Input: dimensioned drawing with shaded views. Units: mm. Origin: part minimum x, y, z. Give positions to 0.01 mm unless a question says otherwise; leave off trailing zeros. Write each loop counter-clockwise with the first axis right and the second up, starting at its lowest first coordinate (ties: lowest second). Pieces come first, ordered by that corner, then holes.
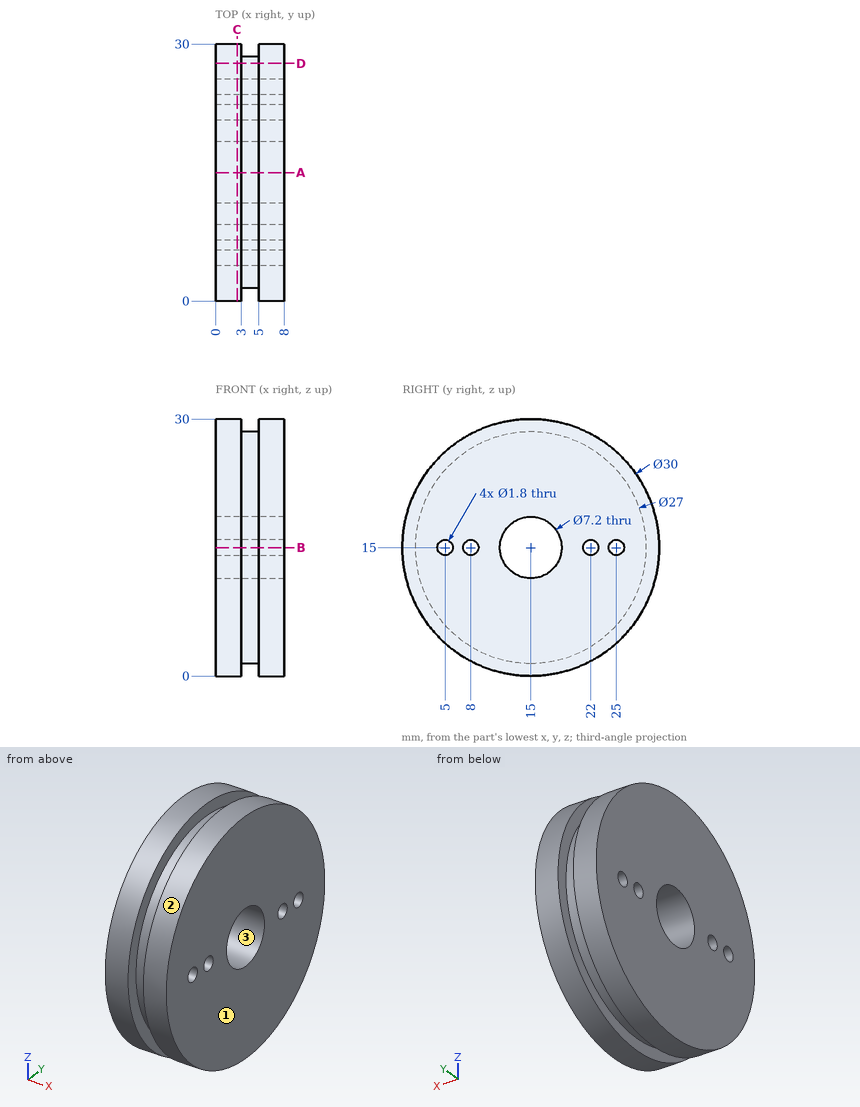
Item 1: Section A-A, the plane y = 15. Return the cut outline in (x, z), plus the area to 3 significant figures.
Found:
outline: (0, 0) - (3, 0) - (3, 1.5) - (5, 1.5) - (5, 0) - (8, 0) - (8, 11.4) - (0, 11.4) - close; (0, 18.6) - (8, 18.6) - (8, 30) - (5, 30) - (5, 28.5) - (3, 28.5) - (3, 30) - (0, 30) - close
area: 176 mm2
Item 2: Pull-direction query (Z, two-part tool) for the marked faces 1, 2 and 3; classes: +Z half, -Z half, draft (parallel to the pull), parting line (faces both ways), or undercut.
Found:
face 1: draft
face 2: parting line
face 3: undercut
Item 3: Section C-C, the plane x = 2.5. Return the cut outline in (y, z), plus the area to 3 significant figures.
Found:
outline: circle Ø30 at (15, 15); hole circle Ø1.8 at (5, 15); hole circle Ø1.8 at (8, 15); hole circle Ø7.2 at (15, 15); hole circle Ø1.8 at (22, 15); hole circle Ø1.8 at (25, 15)
area: 656 mm2
Item 4: Section D-D, the plane y = 27.75. Return the cut outline in (x, z), plus the area to 3 significant figures.
Found:
outline: (0, 7.1) - (3, 7.1) - (3, 10.56) - (5, 10.56) - (5, 7.1) - (8, 7.1) - (8, 22.9) - (5, 22.9) - (5, 19.44) - (3, 19.44) - (3, 22.9) - (0, 22.9) - close
area: 113 mm2
Item 5: Line query: L1, parallel to Y at x = 6, z = 15; L2, parallel to Y at x = 4.25, z = 15; L3, parallel to Z at x = 7, y = 15. Output: solid intervals per line, ascending.
Found:
L1: y = 0 to 4.1, 5.9 to 7.1, 8.9 to 11.4, 18.6 to 21.1, 22.9 to 24.1, 25.9 to 30
L2: y = 1.5 to 4.1, 5.9 to 7.1, 8.9 to 11.4, 18.6 to 21.1, 22.9 to 24.1, 25.9 to 28.5
L3: z = 0 to 11.4, 18.6 to 30
Item 6: Pin query (flat end, axial travel): pin 1 Ø1.4 at (y, z) = (25, 15) entering from +X; pin 2 Ø2 at (x, z) = (5, 24) entering from +Y; pin 3 Ø2 at (x, y) = (4.5, 9.5) entering from +Z; pin 4 Ø4 at (x, z) = (1.5, 20.5) entering from +Y. Return the tip coordinate at first contact, or that it passes through.
Found:
pin 1: passes through
pin 2: stops at y = 27.69
pin 3: stops at z = 29.27
pin 4: stops at y = 29.59
Item 7: Section B-B, the plane z = 15. State how many separate pieces and enclosed holes the cut face has, plus the area to 3 significant figures.
Found:
separate pieces: 6
enclosed holes: 0
area: 119 mm2
